Geometry: final body of the model. Coordinates: model frame, mm. Round coordinates to 2 decimals unless told otherwise and drop trailing zeros. Loops run counter-clockwise (first coordinate to the right, second up) from the corner with the lowest first, then second, coordinate; pieces in that order, holes last. Notation, with made-up numbers: (70, 67.5) -> (113, 67.5) arc R20 cw to (113, 74.5) -> close; hole circle Ø2 at (-5, 39.5). An arc over 180 degrees is marked (long way). Answer in a Markdown table with one row per item.
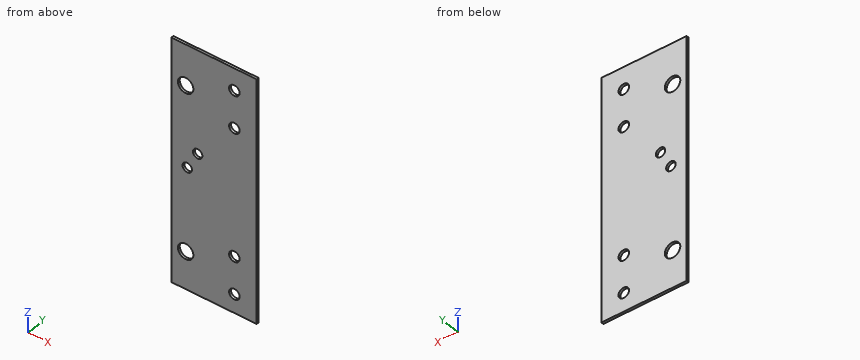
```python
from build123d import *

# Parameters (mm, degrees)
SKETCH1_R           = 5.207
SKETCH1_R_2         = 3.556
BOSS_EXTRUDE1_DEPTH = 1.5875
SKETCH2_R           = 3.175
CUT_EXTRUDE1_DEPTH  = 2.5875
SKETCH3_R           = 3.175
CUT_EXTRUDE2_DEPTH  = 2.5875


with BuildPart() as part:
    # Sketch1 → Boss-Extrude1 (new body)
    with BuildSketch(Plane(origin=(0, 0, 0), x_dir=(1, 0, 0), z_dir=(0, 1, 0))):
        Polygon((-28.60675, 81.407), (28.60675, 81.407), (28.60675, -81.407), (28.60675, -83.693), (-28.60675, -83.693), (-28.60675, -81.407), align=None)
        with Locations((-19.08175, 56.007)):
            Circle(SKETCH1_R, mode=Mode.SUBTRACT)
        with Locations((-19.08175, -56.007)):
            Circle(SKETCH1_R, mode=Mode.SUBTRACT)
        with Locations((13.62075, 68.707)):
            Circle(SKETCH1_R_2, mode=Mode.SUBTRACT)
        with Locations((13.62075, 43.307)):
            Circle(SKETCH1_R_2, mode=Mode.SUBTRACT)
        with Locations((13.62075, -43.307)):
            Circle(SKETCH1_R_2, mode=Mode.SUBTRACT)
        with Locations((13.62075, -68.707)):
            Circle(SKETCH1_R_2, mode=Mode.SUBTRACT)
    extrude(amount=BOSS_EXTRUDE1_DEPTH)

    # Sketch2 → Cut-Extrude1 (cut, through all)
    with BuildSketch(Plane(origin=(0, 1.5875, 0), x_dir=(1, 0, 0), z_dir=(0, 1, 0))):
        with Locations((-17.992815678, -1.143)):
            Circle(SKETCH2_R)
    extrude(amount=-CUT_EXTRUDE1_DEPTH, mode=Mode.SUBTRACT)

    # Sketch3 → Cut-Extrude2 (cut, through all)
    with BuildSketch(Plane.XZ):
        with Locations((-11.01725, 13.843)):
            Circle(SKETCH3_R)
    extrude(amount=-CUT_EXTRUDE2_DEPTH, mode=Mode.SUBTRACT)


solid = part.part
```
Item 1: Section query B-B, the plane y = 1.3. State how many separate pieces and enclosed holes the cut face has, and give its area (3 significant figures).
Ans:
| item | result |
|---|---|
| separate pieces | 1 |
| enclosed holes | 8 |
| area | 9,050 mm2 |
Item 2: First-contact query: P1, Ø8.5, axis at x = -17.99, z = 1.14, coming from the -Y side. Flat tip, straight axial feed; report the tip coordinate or a pass-through.
Ans:
| item | result |
|---|---|
| P1 | y = 0 |
Item 3: Ray query, L1, parallel to Z at x = 13.5, y = 1.4; L2, parallel to Z at x = 16.5, y = 1.15; L3, parallel to X at y = 1, z = 13. Return the intervals inside material, ascending.
Ans:
| item | result |
|---|---|
| L1 | -81.41 to -72.26, -65.15 to -46.86, -39.75 to 39.75, 46.86 to 65.15, 72.26 to 83.69 |
| L2 | -81.41 to -70.79, -66.62 to -45.39, -41.22 to 41.22, 45.39 to 66.62, 70.79 to 83.69 |
| L3 | -28.61 to -14.08, -7.96 to 28.61 |
Item 4: Section query A-A, the plane x = -19. Output: boundary loops of the cut face in (y, z).
Ans:
| item | result |
|---|---|
| outline | (0, -81.41) -> (1.59, -81.41) -> (1.59, -61.21) -> (0, -61.21) -> close; (0, -50.8) -> (1.59, -50.8) -> (1.59, -1.87) -> (0, -1.87) -> close; (0, 4.15) -> (1.59, 4.15) -> (1.59, 50.8) -> (0, 50.8) -> close; (0, 61.21) -> (1.59, 61.21) -> (1.59, 83.69) -> (0, 83.69) -> close |
